from build123d import *

# Parameters (mm, degrees)
SKETCH1_R           = 4.748524974
SKETCH1_R_2         = 2.967828109
BOSS_EXTRUDE1_DEPTH = 3.175
BOSS_EXTRUDE2_DEPTH = 25.4


with BuildPart() as part:
    # Sketch1 → Boss-Extrude1 (new body)
    with BuildSketch(Plane(origin=(0, 0, 0), x_dir=(1, 0, 0), z_dir=(0, 1, 0))):
        with BuildLine():
            Line((-12.535412203, -0.532735955), (-12.641288389, -15.698136108))
            Line((-12.641288389, -15.698136108), (-16.451288389, -15.698136108))
            Line((-16.451288389, -15.698136108), (-16.451288389, 20.814363892))
            Line((-16.451288389, 20.814363892), (34.348711611, 20.814363892))
            Line((34.348711611, 20.814363892), (34.348711611, -15.698136108))
            Line((34.348711611, -15.698136108), (-9.725725357, -15.698136108))
            Line((-9.725725357, -15.698136108), (-9.725725357, -0.458136108))
            ThreePointArc((-9.725725357, -0.458136108), (-11.278719551, 5.08443165), (-12.535412203, -0.532735955))
        make_face()
        with Locations(Location((3.061154267, 2.126474445, 0), (0, 0, 270))):
            Circle(SKETCH1_R, mode=Mode.SUBTRACT)
        with Locations(Location((10.183941728, 14.463504219, 0), (0, 0, 270))):
            Circle(SKETCH1_R_2, mode=Mode.SUBTRACT)
        with Locations(Location((10.183941728, -10.210555329, 0), (0, 0, 270))):
            Circle(SKETCH1_R_2, mode=Mode.SUBTRACT)
    extrude(amount=BOSS_EXTRUDE1_DEPTH)

    # Sketch2 → Boss-Extrude2 (add)
    with BuildSketch(Plane.XZ):
        with BuildLine():
            Line((20.263560728, -20.814363892), (34.348711611, -20.814363892))
            Line((34.348711611, -20.814363892), (34.348711611, 15.698136108))
            Line((34.348711611, 15.698136108), (21.156547566, 15.698136108))
            ThreePointArc((21.156547566, 15.698136108), (28.453561223, -2.747496977), (20.263560728, -20.814363892))
        make_face()
    extrude(amount=BOSS_EXTRUDE2_DEPTH)


solid = part.part
The model under review builds one solid part; all positions refer to its coordinate system, in mm. A direction names the side the tool comes from. Give positions to 0.01 mm unless a question says otherwise; leave off trailing zeros. Order: outer loops, then holes, each group sorted by start corner. A loop starts at its lowest first (then second) coordinate and runs counter-clockwise, first axis right, second up. Notation, with made-up numbers: M -16,87 L 4,87 A20 cw 4,103 Z; hole C 32.5,47 d5. An arc over 180 degrees is marked long. Answer in a Markdown table with one row per item. Add a question column.
1. Mouldability with a two-part tool opening along X and no side actions: class faces 1 (the cylindrical face through (-11.169, 1.565, -5.085)), 2 (the flat face through (34.349, -11, -3)), 3 (the flat face through (22, -9, -20.814)) as released by +X, released by -X, zero draft, split by the parting line, or undercut.
2. Add section D-D on y = -12.5. State the section outline as (x, z) points, plus the area to 3 significant figures.
3. Add section C-C on z = -13.5. State the section outline as (x, y) points (3 decimals), plus the area to 3 significant figures.
4. Add section A-A on z = 11. State the section outline as (x, y) points (3 decimals).
5. For pin 1 Ø2 at (x, z) = (14, -3.5) entering from -Y; pin 2 Ø4 at (y, z) = (-13, -8.5) entering from -X; pin 3 Ø1.5 at (y, z) = (-21.5, 7) entering from -X, all flat-tipped, find the tip position at first contact; note any pin that passes through.
6. Add section B-B on x = 5.5. State the section outline as (y, z) points (3 decimals), plus the area to 3 significant figures.
7. Machinability: for faces 4 (the flat face through (-9.726, 2, 8)), 5 (the flat face through (30, -25.4, -2)), 6 (the flat face through (6, 0, -7)), which of the approach directions +Z, -Z, +X, -X, +Y, -Y give a long, thin tool a straight path to every point of the face, cutting with its end or side? Answer none if there is none.
8. To check wall thickness, follow line 1 along Y through (x, z) = (-4, -9) (3 decimals); line 2 along X through (y, z) = (-16.75, 13); line 3 along Z through (x, y) = (23.5, -20.25). State the ranges of each line that lie inside material, in increasing order.
The answers:
| question | item | result |
|---|---|---|
| 1 | face 1 | undercut |
| 1 | face 2 | released by +X |
| 1 | face 3 | zero draft |
| 2 | outline | M 20.26,-20.81 L 34.35,-20.81 L 34.35,15.7 L 21.16,15.7 A25.4 cw Z |
| 2 | area | 303 mm2 |
| 3 | outline | M -16.451,0 L 7.377,0 L 7.377,3.175 L -16.451,3.175 Z; M 12.991,0 L 25.772,0 L 25.772,-25.4 L 34.349,-25.4 L 34.349,3.175 L 12.991,3.175 Z |
| 3 | area | 361 mm2 |
| 4 | outline | M -16.451,0 L -12.608,0 L -12.608,3.175 L -16.451,3.175 Z; M -9.726,0 L 7.323,0 L 7.323,3.175 L -9.726,3.175 Z; M 13.045,0 L 24.806,0 L 24.806,-25.4 L 34.349,-25.4 L 34.349,3.175 L 13.045,3.175 Z |
| 5 | pin 1 | y = 0 |
| 5 | pin 2 | x = 27.04 |
| 5 | pin 3 | x = 26.46 |
| 6 | outline | M 0,-20.814 L 3.175,-20.814 L 3.175,-6.201 L 0,-6.201 Z; M 0,1.948 L 3.175,1.948 L 3.175,15.698 L 0,15.698 Z |
| 6 | area | 90.1 mm2 |
| 7 | face 4 | +Z, +Y, -Y |
| 7 | face 5 | +Z, -Z, +X, -X, -Y |
| 7 | face 6 | -X, -Y |
| 8 | line 1 | 0 to 3.175 |
| 8 | line 2 | 23.47 to 34.35 |
| 8 | line 3 | -20.81 to -17.21, 12.95 to 15.7 |
